from build123d import *

# Parameters (mm, degrees)
F0_R     = 38.1
F1_DEPTH = 4
F2_R     = 4.5
F2_W     = 8
F2_H     = 8
F3_DEPTH = 4.001
F2_W_2   = 7.2
F2_H_2   = 7.2
F4_DEPTH = 12
F2_R_2   = 6
F5_DEPTH = 4
F6_W     = 1.8
F6_H     = 18.1
F6_W_2   = 18.1
F6_H_2   = 1.8
F7_DEPTH = 2


with BuildPart() as f1:
    # F0 (on Top) → F1 (new body)
    with BuildSketch(Plane.XY):
        Circle(F0_R)
    extrude(amount=F1_DEPTH)

    # F2 (on face) → F3 (cut, through all)
    with BuildSketch(Plane.XY.offset(4)):
        Circle(F2_R)
        with Locations((0, 12)):
            Rectangle(F2_W, F2_H)
        with Locations((0, -12)):
            Rectangle(F2_W, F2_H)
    extrude(amount=-F3_DEPTH, mode=Mode.SUBTRACT)

    # F2 (on face) → F4 (join)
    with BuildSketch(Plane.XY.offset(4)):
        with Locations((12, 0)):
            Rectangle(F2_W_2, F2_H_2)
        with Locations((-12, 0)):
            Rectangle(F2_W_2, F2_H_2)
    extrude(amount=F4_DEPTH)

    # F2 (on face) → F5 (join)
    with BuildSketch(Plane.XY.offset(4)):
        Circle(F2_R_2)
        Circle(F2_R, mode=Mode.SUBTRACT)
    extrude(amount=F5_DEPTH)

    # F6 (on face) → F7 (cut)
    with BuildSketch(Plane.XY.offset(4)):
        with Locations((0, 27.05)):
            Rectangle(F6_W, F6_H)
        with Locations((-27.05, 0)):
            Rectangle(F6_W_2, F6_H_2)
        with Locations((0, -27.05)):
            Rectangle(F6_W, F6_H)
        with Locations((27.05, 0)):
            Rectangle(F6_W_2, F6_H_2)
    extrude(amount=-F7_DEPTH, mode=Mode.SUBTRACT)


solid = f1.part
Geometry: final body of the model. Coordinates: model frame, mm. A direction names the side the tool comes from. Give positions to 0.01 mm unless a question says otherwise; leave off trailing zeros. Write each loop counter-clockwise with the first axis right and the second up, starting at its lowest first coordinate (ties: lowest second). Pieces come first, ordered by that corner, then holes. Notation, with made-up numbers: (63.5, 42.5) -> (116.5, 42.5) arc R19 cw to (116.5, 46.5) -> close; hole circle Ø1 at (76, 40). An arc over 180 degrees is marked (long way). Answer in a Markdown table with one row per item.
(1) Section query C-C on z = 12.25. Return loops of the section in (x, y).
Answers below:
| item | result |
|---|---|
| outline | (-15.6, -3.6) -> (-8.4, -3.6) -> (-8.4, 3.6) -> (-15.6, 3.6) -> close; (8.4, -3.6) -> (15.6, -3.6) -> (15.6, 3.6) -> (8.4, 3.6) -> close |
(2) Section query B-B on y = 0. Return loops of the section in (x, z), then the cut area to 3 significant figures.
Answers below:
| item | result |
|---|---|
| outline | (-38.1, 0) -> (-4.5, 0) -> (-4.5, 8) -> (-6, 8) -> (-6, 4) -> (-8.4, 4) -> (-8.4, 16) -> (-15.6, 16) -> (-15.6, 4) -> (-18, 4) -> (-18, 2) -> (-36.1, 2) -> (-36.1, 4) -> (-38.1, 4) -> close; (4.5, 0) -> (38.1, 0) -> (38.1, 4) -> (36.1, 4) -> (36.1, 2) -> (18, 2) -> (18, 4) -> (15.6, 4) -> (15.6, 16) -> (8.4, 16) -> (8.4, 4) -> (6, 4) -> (6, 8) -> (4.5, 8) -> close |
| area | 381 mm^2 |
(3) Section query A-A on x = 0. Return loops of the section in (y, z).
Answers below:
| item | result |
|---|---|
| outline | (-38.1, 0) -> (-16, 0) -> (-16, 4) -> (-18, 4) -> (-18, 2) -> (-36.1, 2) -> (-36.1, 4) -> (-38.1, 4) -> close; (-8, 0) -> (-4.5, 0) -> (-4.5, 8) -> (-6, 8) -> (-6, 4) -> (-8, 4) -> close; (4.5, 0) -> (8, 0) -> (8, 4) -> (6, 4) -> (6, 8) -> (4.5, 8) -> close; (16, 0) -> (38.1, 0) -> (38.1, 4) -> (36.1, 4) -> (36.1, 2) -> (18, 2) -> (18, 4) -> (16, 4) -> close |
(4) Section query D-D on x = -25.5. Return loops of the section in (y, z), then the cut area to 3 significant figures.
Answers below:
| item | result |
|---|---|
| outline | (-28.31, 0) -> (28.31, 0) -> (28.31, 4) -> (0.9, 4) -> (0.9, 2) -> (-0.9, 2) -> (-0.9, 4) -> (-28.31, 4) -> close |
| area | 223 mm^2 |
(5) Set-up query: faces 4 (the flat face through (8.4, 0, 10)), 5 (the flat face through (0, 8, 2)), 6 (the flat face through (27, 0, 2)). Return all of +Z, -Z, +X, -X, +Y, -Y with unobstructed straight access to the full face (end or side cutting, diameter ignored); none if empty.
Answers below:
| item | result |
|---|---|
| face 4 | +Z, +Y, -Y |
| face 5 | +Z, -Z |
| face 6 | +Z |
(6) Draft query along Y for faces 1 (the flat face through (0, -8, 2)), 2 (the cylindrical face through (-6, 0, 6)), 3 (the flat face through (12, 0, 16)). Return one class per face: +Y half, -Y half, draft (parallel to the pull), parting line (faces both ways), or undercut.
Answers below:
| item | result |
|---|---|
| face 1 | undercut |
| face 2 | parting line |
| face 3 | draft |
(7) Ray query, line 1 along Y through (x, z) = (0, 1.2); line 2 along Y through (x, z) = (0, 2.2); line 3 along Y through (x, z) = (0, 5). Return the intervals inside material, ascending. Write a range as [from, to].
Answers below:
| item | result |
|---|---|
| line 1 | [-38.1, -16], [-8, -4.5], [4.5, 8], [16, 38.1] |
| line 2 | [-38.1, -36.1], [-18, -16], [-8, -4.5], [4.5, 8], [16, 18], [36.1, 38.1] |
| line 3 | [-6, -4.5], [4.5, 6] |
(8) Pin query (flat end, axial travel): pin 1 (3 mm diameter, centred on y = -10.5, z = 3, fed in from +X); pin 2 (1.6 mm diameter, centred on x = -26.5, z = 2.5, fed in from +Y); pin 3 (1.2 mm diameter, centred on y = 11, z = 2, fed in from +X); pin 4 (5 mm diameter, centred on y = -18.5, z = 7.5, fed in from -X). Return the tip coordinate at first contact, or that it passes through.
Answers below:
| item | result |
|---|---|
| pin 1 | x = 37.02 |
| pin 2 | y = 28.13 |
| pin 3 | x = 36.65 |
| pin 4 | through |
